```python
from build123d import *

# Parameters (mm, degrees)
ESQUISSE1_W             = 68.2
ESQUISSE1_H             = 38.8
BOSS_EXTRU_2_DEPTH      = 15
ESQUISSE3_W             = 10
ESQUISSE3_H             = 6
ENL_V_MAT_EXTRU_1_DEPTH = 2
ESQUISSE4_R             = 1.75
ENL_V_MAT_EXTRU_2_DEPTH = 80.885417943
ESQUISSE6_W             = 6
ESQUISSE6_H             = 6
ENL_V_MAT_EXTRU_3_DEPTH = 10


with BuildPart() as part:
    # Esquisse1 → Boss.-Extru.2 (new body)
    with BuildSketch(Plane.XY):
        with Locations((34.1, 19.4)):
            Rectangle(ESQUISSE1_W, ESQUISSE1_H)
    extrude(amount=BOSS_EXTRU_2_DEPTH)

    # Esquisse3 → Enlèv. mat.-Extru.1 (cut)
    with BuildSketch(Plane.XY.offset(15)):
        with Locations((5, 35.8)):
            Rectangle(ESQUISSE3_W, ESQUISSE3_H)
        with Locations((5, 3)):
            Rectangle(ESQUISSE3_W, ESQUISSE3_H)
        with Locations((63.2, 3)):
            Rectangle(ESQUISSE3_W, ESQUISSE3_H)
        with Locations((63.2, 35.8)):
            Rectangle(ESQUISSE3_W, ESQUISSE3_H)
    extrude(amount=-ENL_V_MAT_EXTRU_1_DEPTH, mode=Mode.SUBTRACT)

    # Esquisse4 → Enlèv. mat.-Extru.2 (cut, through all)
    with BuildSketch(Plane.XY.offset(15)):
        with Locations((3, 35.8)):
            Circle(ESQUISSE4_R)
        with Locations((3, 3)):
            Circle(ESQUISSE4_R)
        with Locations((65.2, 35.8)):
            Circle(ESQUISSE4_R)
        with Locations((65.2, 3)):
            Circle(ESQUISSE4_R)
    extrude(amount=-ENL_V_MAT_EXTRU_2_DEPTH, mode=Mode.SUBTRACT)

    # Esquisse6 → Enlèv. mat.-Extru.3 (cut)
    with BuildSketch(Plane(origin=(0, 0, 0), x_dir=(-1, 0, 0), z_dir=(0, 0, -1))):
        with Locations((-65.2, 35.8)):
            Rectangle(ESQUISSE6_W, ESQUISSE6_H)
        with Locations((-3, 35.8)):
            Rectangle(ESQUISSE6_W, ESQUISSE6_H)
        with Locations((-3, 3)):
            Rectangle(ESQUISSE6_W, ESQUISSE6_H)
        with Locations((-65.2, 3)):
            Rectangle(ESQUISSE6_W, ESQUISSE6_H)
    extrude(amount=-ENL_V_MAT_EXTRU_3_DEPTH, mode=Mode.SUBTRACT)


solid = part.part
```
Read the model definition and answer for the solid it produces. Units are mm, in the model's axes. A direction names the side the tool comes from. Coordinates: 2 decimals unless noted, no trailing zeros. Loops run counter-clockwise (first coordinate to the right, second up) from the corner with the lowest first, then second, coordinate; pieces in that order, holes last. Notation, with made-up numbers: (13, 55.25) - (34, 55.25) arc R19 ccw to (34, 64.25) - close; hole circle Ø5 at (-36.5, 27.5). An arc over 180 degrees is marked (long way). Answer in a Markdown table with one row per item.
1. Which of the six approach directions +Z, -Z, +X, -X, +Y, -Y give full straight-line access (tool end or side, diameter ignored) to faces 1 (the face through (65, 32.8, 5)), 2 (the face through (6, 3, 5)), 3 (the face through (4.4, 37.2, 10))?
Conclusion:
| item | result |
|---|---|
| face 1 | -Z, +X, +Y |
| face 2 | -Z, -X, -Y |
| face 3 | -Z, -X, +Y |
2. Given pin 1 (1.8 mm diameter, centred on x = 1.5, y = 35.5, fed in from -Z); pin 2 (1 mm diameter, centred on x = 7.5, z = 14, fed in from +Y); pin 3 (3 mm diameter, centred on x = 64, z = 7, fed in from -Y), each flat-ended and moving along its own axis, determine where each tip first touches the part or whether it passes through.
Conclusion:
| item | result |
|---|---|
| pin 1 | stops at z = 10 |
| pin 2 | stops at y = 32.8 |
| pin 3 | stops at y = 6 |
3. Find section B-B, the plane x = 3. Write down the section's boundary in (y, z).
Conclusion:
| item | result |
|---|---|
| outline | (0, 10) - (1.25, 10) - (1.25, 13) - (0, 13) - close; (4.75, 10) - (6, 10) - (6, 0) - (32.8, 0) - (32.8, 10) - (34.05, 10) - (34.05, 13) - (32.8, 13) - (32.8, 15) - (6, 15) - (6, 13) - (4.75, 13) - close; (37.55, 10) - (38.8, 10) - (38.8, 13) - (37.55, 13) - close |
4. Straight lines are drawn through the part: line 1 (Y direction, x = 65.2, z = 10.8); line 2 (Y direction, x = 4, z = 11.75); line 3 (X direction, y = 36, z = 9). For each, find the intervals that lie inside material, in ascending order.
Conclusion:
| item | result |
|---|---|
| line 1 | y = 0 to 1.25, 4.75 to 34.05, 37.55 to 38.8 |
| line 2 | y = 0 to 1.56, 4.44 to 34.36, 37.24 to 38.8 |
| line 3 | x = 6 to 62.2 |
5. Determine the mould class of faces 4 (the face through (5, 6, 14)), 5 (the face through (63.81, 1.94, 11.52)), 6 (the face through (62.2, 3, 5)), 7 (the face through (6, 36, 5)) for opening direction X: +X half, -X half, draft (parallel to the pull), parting line (faces both ways), or undercut.
Conclusion:
| item | result |
|---|---|
| face 4 | draft |
| face 5 | undercut |
| face 6 | +X half |
| face 7 | -X half |
6. Find section A-A, the plane y = 3. Write down the section's boundary in (x, z), then the cut area to 3 significant figures.
Conclusion:
| item | result |
|---|---|
| outline | (0, 10) - (1.25, 10) - (1.25, 13) - (0, 13) - close; (4.75, 10) - (6, 10) - (6, 0) - (62.2, 0) - (62.2, 10) - (63.45, 10) - (63.45, 13) - (58.2, 13) - (58.2, 15) - (10, 15) - (10, 13) - (4.75, 13) - close; (66.95, 10) - (68.2, 10) - (68.2, 13) - (66.95, 13) - close |
| area | 842 mm² |
